The model under review builds one solid part; all positions refer to its coordinate system, in mm. Face numbers are marked on the shaded views. A direction names the side the tool comes from. Give positions to 0.01 mm unless a question says otherwise; leave off trailing zeros. Loops run counter-clockwise (first coordinate to the right, second up) from the corner with the lowest first, then second, coordinate; pieces in that order, holes last. Notation, with made-up numbers: M -4,-1.75 L 16,-1.75 A13 ccw 16,5.25 Z; hole C -9,12.25 d7. An arc over 180 degrees is marked long. Put each result on its own line as item: value. Start each with the question number.
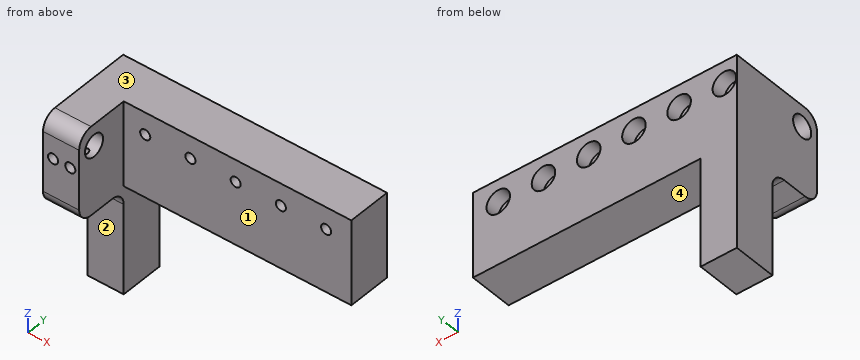
Autodesk Inventor part; units mm, degrees
ref_plane "YZ Plane" through (0, 0, 0) normal (1, 0, 0) x (0, 1, 0)
ref_plane "XZ Plane" through (0, 0, 0) normal (0, 1, 0) x (-1, 0, 0)
ref_plane "XY Plane" through (0, 0, 0) normal (0, 0, 1) x (1, 0, 0)
ref_plane "Work Plane1" through (18, 18.5, -30) normal (0, 1, 0) x (0, 0, -1)
sketch "Sketch1" plane through (18, 18.5, -30) normal (0, 1, 0) x (0, 0, -1)
  line L0 (-30.1565, -29.8905) -> (-15.0465, -29.8905) construction
  line L1 (-30, -38) -> (-30, 18) construction
  circle A0 centre (-25, -20) radius 1.45 construction
  circle A1 centre (25, -20) radius 1.45 construction
  circle A2 centre (25, 0) radius 1.45 construction
  circle A3 centre (-25, 0) radius 1.45 construction
  circle A4 centre (10, -35) radius 1.45 construction
  circle A5 centre (10, 15) radius 1.45 construction
  circle A6 centre (-10, 15) radius 1.45 construction
  circle A7 centre (-10, -35) radius 1.45 construction
  circle A8 centre (25, 15) radius 2.325 construction
  circle A9 centre (-25, -35) radius 2.325 construction
  circle A10 centre (25, -35) radius 2.325 construction
  circle A11 centre (-25, 15) radius 2.325 construction
  line L2 (-28, 20) -> (-30, 18) construction
  line L3 (-28, 20) -> (28, 20) construction
  line L4 (30, 18) -> (28, 20) construction
  line L5 (30, 18) -> (30, -38) construction
  line L6 (28, -40) -> (30, -38) construction
  line L7 (28, -40) -> (-28, -40) construction
  line L8 (-30, -38) -> (-28, -40) construction
  line L9 (-30, -38) -> (-30, 18) construction
  circle A12 centre (17.5, -27.5) radius 1.95 construction
  circle A13 centre (-17.5, 7.5) radius 1.95 construction
  circle A14 centre (-17.5, -27.5) radius 1.95 construction
  circle A15 centre (17.5, 7.5) radius 1.95 construction
  circle A16 centre (0, -10) radius 7.5 construction
  line L10 (-0.1565, 20) -> (-30.1565, 20)
  line L11 (-30.1565, 20) -> (-30.1565, 30)
  line L12 (-30.1565, 30) -> (-0.1565, 30)
  line L13 (-0.1565, 30) -> (-0.1565, 20)
  line L14 (-30.1565, 30) -> (-53.7065, 30)
  line L15 (-53.7065, 30) -> (-53.7065, -42.9244)
  line L16 (-53.7065, -42.9244) -> (-30.1565, -42.9244)
  line L17 (-30.1565, -42.9244) -> (-30.1565, 30)
  circle A17 centre (-47.5565, 1.5545) radius 1.75 construction
  circle A18 centre (-47.5565, -10.9455) radius 1.75 construction
  circle A19 centre (-47.5565, -23.4455) radius 1.75 construction
  circle A20 centre (-47.5565, -35.9455) radius 1.75 construction
  line L18 (-41.6065, -40.3471) -> (-53.7065, -40.3471) construction
  line L19 (-41.6065, -40.3471) -> (-41.6065, 9.6529) construction
  line L20 (-41.6065, 9.6529) -> (-53.7065, 9.6529) construction
  line L21 (-53.7065, -40.3471) -> (-53.7065, 9.6529) construction
  circle A21 centre (-47.5565, -48.4455) radius 1.75 construction
  circle A22 centre (-47.5565, -60.9455) radius 1.75 construction
  circle A23 centre (-47.5565, -73.4455) radius 1.75 construction
  circle A24 centre (-47.5565, -85.9455) radius 1.75 construction
  line L22 (-41.6065, -90.3471) -> (-53.7065, -90.3471) construction
  line L23 (-41.6065, -90.3471) -> (-41.6065, -40.3471) construction
  line L24 (-41.6065, -40.3471) -> (-53.7065, -40.3471) construction
  line L25 (-53.7065, -90.3471) -> (-53.7065, -40.3471) construction
  point P0 (-30.1565, 20)
  dimension "d0" = 10
  dimension "d1" = 30
extrude "Extrusion1" add sketch "Sketch1" against normal blind 12
sketch "Sketch2" plane through (18, 18.5, -30) normal (0, 1, 0) x (1, 0, 0)
  circle A0 centre (35.9455, -47.5565) radius 1.75
  point P0 (-18, -30)
hole "Hole1" at (53.9455, 18.5, 17.5565) direction (0, -1, 0) diameter 2.8 end through all counterbore diameter 6.5 counterbore depth 4
pattern_linear "Rectangular Pattern1" count 9 spacing 12.5 along (-1, 0, 0) of "Hole1"
sketch "Sketch3" plane through (18, 6.5, -30) normal (0, -1, 0) x (1, 0, 0)
  line L0 (-30, 53.7065) -> (-30, 0.1565)
  line L1 (-30, 0.1565) -> (-20, 0.1565)
  line L2 (-20, 0.1565) -> (-20, 30.1565)
  line L3 (-20, 30.1565) -> (42.9244, 30.1565)
  line L4 (42.9244, 30.1565) -> (42.9244, 53.7065)
  line L5 (42.9244, 53.7065) -> (-30, 53.7065)
  line L6 (-30, 53.7065) -> (42.9244, 53.7065)
  line L7 (-30, 53.7065) -> (-20, 53.7065)
  line L8 (-20, 53.7065) -> (-20, 29.1031)
  line L9 (-20, 29.1031) -> (-30, 29.1031)
  line L10 (-30, 29.1031) -> (-30, 53.7065)
  point P0 (-18, 30)
  point P1 (-30, 29.1031)
  dimension "d14" = 10
extrude "Extrusion2" add sketch "Sketch3" along normal blind 15 contours L5 L8 L2 L9 L0
sketch "Sketch4" plane through (-12, 18.5, -29.8435) normal (-1, 0, 0) x (0, 0, 1)
  line L0 (0, 0) -> (53.55, 0)
  line L1 (0, 0) -> (0, -12)
  line L2 (28.9466, -12) -> (0, -12)
  line L3 (28.9466, -12) -> (28.9466, -27)
  line L4 (53.55, -27) -> (28.9466, -27)
  line L5 (53.55, 0) -> (53.55, -27)
  circle A0 centre (40.6, -17.5571) radius 2.1
  circle A1 centre (47.6565, -22.005) radius 1.6829
  arc A2 (53.5014, -16.3734) -> (53.6565, -16.1421) centre (53.4065, -16.1421) ccw construction
  arc A3 (53.5014, -16.3734) -> (52.9237, -16.8727) centre (53.9565, -17.4838) ccw construction
  arc A4 (52.7304, -16.9945) -> (52.9237, -16.8727) centre (52.7086, -16.7455) ccw construction
  line L6 (52.7304, -16.9945) -> (52.3847, -17.0247) construction
  arc A5 (52.3847, -17.0247) -> (52.1565, -17.2738) centre (52.4065, -17.2738) ccw construction
  line L7 (52.1565, -17.2738) -> (52.1565, -17.7262) construction
  arc A6 (52.1565, -17.7262) -> (52.3847, -17.9753) centre (52.4065, -17.7262) ccw construction
  line L8 (52.3847, -17.9753) -> (52.7513, -18.0073) construction
  arc A7 (52.9411, -18.1232) -> (52.7513, -18.0073) centre (52.7295, -18.2564) ccw construction
  arc A8 (52.9411, -18.1232) -> (53.5014, -18.5941) centre (53.9565, -17.4838) ccw construction
  arc A9 (53.6565, -18.8254) -> (53.5014, -18.5941) centre (53.4065, -18.8254) ccw construction
  line L9 (53.6565, -18.8254) -> (53.6565, -19.5) construction
  line L10 (53.6565, -19.5) -> (53.1565, -20) construction
  line L11 (53.1565, -20) -> (42.1566, -20) construction
  line L12 (42.1566, -20) -> (41.6566, -19.5) construction
  line L13 (41.6566, -19.5) -> (41.6566, -18.8254) construction
  arc A10 (41.8117, -18.5941) -> (41.6566, -18.8254) centre (41.9066, -18.8254) ccw construction
  arc A11 (41.8117, -18.5941) -> (42.372, -18.1232) centre (41.3566, -17.4838) ccw construction
  arc A12 (42.5618, -18.0073) -> (42.372, -18.1232) centre (42.5836, -18.2564) ccw construction
  line L14 (42.5618, -18.0073) -> (42.9283, -17.9753) construction
  arc A13 (42.9283, -17.9753) -> (43.1566, -17.7262) centre (42.9066, -17.7262) ccw construction
  line L15 (43.1566, -17.7262) -> (43.1566, -17.2738) construction
  arc A14 (43.1566, -17.2738) -> (42.9283, -17.0247) centre (42.9066, -17.2738) ccw construction
  line L16 (42.9283, -17.0247) -> (42.5827, -16.9945) construction
  arc A15 (42.3894, -16.8727) -> (42.5827, -16.9945) centre (42.6045, -16.7455) ccw construction
  arc A16 (42.3894, -16.8727) -> (41.8117, -16.3734) centre (41.3566, -17.4838) ccw construction
  arc A17 (41.6566, -16.1421) -> (41.8117, -16.3734) centre (41.9066, -16.1421) ccw construction
  line L17 (41.6566, -16.1421) -> (41.6566, -15) construction
  line L18 (41.6566, -15) -> (35.0566, -15) construction
  line L19 (35.0566, -15) -> (34.4566, -15.6) construction
  line L20 (34.4566, -15.6) -> (34.4566, -23.4) construction
  line L21 (34.4566, -23.4) -> (35.6565, -24.6) construction
  line L22 (35.6565, -24.6) -> (59.6565, -24.6) construction
  line L23 (59.6565, -24.6) -> (60.8565, -23.4) construction
  line L24 (60.8565, -23.4) -> (60.8565, -15.6) construction
  line L25 (60.8565, -15.6) -> (60.2565, -15) construction
  line L26 (60.2565, -15) -> (53.6565, -15) construction
  line L27 (53.6565, -15) -> (53.6565, -16.1421) construction
  circle A18 centre (40.7565, -22.005) radius 2.1 construction
  circle A19 centre (54.5565, -22.005) radius 2.1 construction
  point P0 (29.8435, -18.5)
hole "Hole2" at (-12, -3.505, 17.8131) direction (1, 0, 0) diameter 6.1 end through all
fillet "Fillet1" radius 4 3 edges at (-7, -8.5, 23.7065) (-7, -8.5, -0.8969) (-7, 6.5, -0.8969)
sketch "Sketch5" plane through (18, -8.5, -30) normal (0, -1, 0) x (1, 0, 0)
  line L0 (-20, 43.8065) -> (-30, 43.8065) construction
  circle A0 centre (-22.4542, 43.5587) radius 1.4
  circle A1 centre (-27.2211, 43.5587) radius 1.4
  line L1 (-20, 44.7631) -> (-30, 44.7631)
  point P0 (-18, 30)
  dimension "d28" = 2.8
  dimension "d29" = 2.8
extrude "Extrusion3" cut sketch "Sketch5" against normal blind 15
properties part number "30_cellSTORM_UC2_Laser_slider"
(1) We need section C-C, the plane z = 7.5. Write out the cut boundary in (x, y), plus the area to 3 significant figures.
(2) Insertion check: pin 1 (3.5 mm diameter, centred on x = 3.95, z = 17.56, fed in from -Y); pin 2 (4.5 mm diameter, centred on x = 41.45, z = 17.56, fed in from +Y); pin 3 (10 mm diameter, centred on y = 10, z = -6.5, fed in from +X). Each pin has a flat end and moves straight along its axis. Give the tip position at first contact, or say it passes through.
(3) To check wall thickness, follow L1, parallel to Y at x = -8, z = 18; L2, parallel to Y at x = 20.5, z = 22; L3, parallel to Z at x = -4.5, y = 3.25. State the ranges of each line that lie inside material, in increasing order. Write a range as [from, to].
(4) We need section B-B, the plane y = 9.25. Write out the cut boundary in (x, z), plus the area to 3 significant figures.
(5) For the marked faces 1, 2, 3 and 4, list the 3-axis set-ups (+Z, -Z, +X, -X, +Y, -Y) from which the entire face can be reached by the end or side of a thin tool; tool diameter is ignored.
(6) We need section A-A, the plane x = 34.5. Write out the cut boundary in (y, z).
(7) We need section D-D, the plane y = 4. Write out the cut boundary in (x, z).
Check sheet entries:
1. outline: M -12,-8.5 L -2,-8.5 L -2,6.5 L 60.92,6.5 L 60.92,18.5 L -12,18.5 Z
1. area: 1,030 mm²
2. pin 1: stops at y = 6.5
2. pin 2: stops at y = 14.5
2. pin 3: stops at x = -2
3. L1: y = [-8.5, -6.55], [-0.46, 6.5]
3. L2: y = [6.5, 18.5]
3. L3: z = [-0.97, 12.16], [14.96, 23.71]
4. outline: M -12,-29.84 L -2,-29.84 L -2,0.16 L 60.92,0.16 L 60.92,23.71 L -12,23.71 Z; hole C -8.55,17.56 d2.8; hole C 3.95,17.56 d2.8; hole C 16.45,17.56 d2.8; hole C 28.95,17.56 d2.8; hole C 41.45,17.56 d2.8; hole C 53.95,17.56 d2.8
4. area: 1,980 mm²
5. face 1: +Z, -Z, +X, -Y
5. face 2: -Z, +X, -X, -Y
5. face 3: +Z, +X, -X, +Y, -Y
5. face 4: -Z, +X, +Y, -Y
6. outline: M 6.5,0.16 L 18.5,0.16 L 18.5,23.71 L 6.5,23.71 Z
7. outline: M -12,-1.19 L -2,-1.19 L -2,23.71 L -12,23.71 Z; hole C -9.22,13.56 d2.8; hole C -4.45,13.56 d2.8
